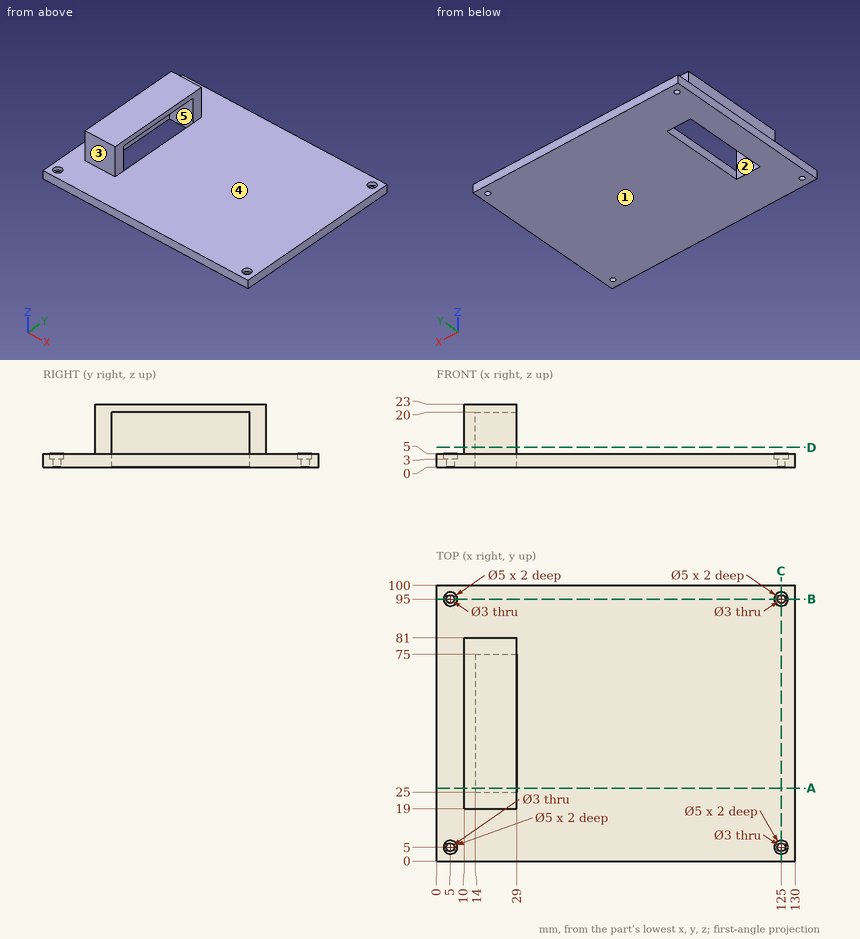
The drawing under review shows one solid part. Ordinate dimensions are in mm from its lowest x, y, z. A direction names the side the tool comes from. Give positions to 0.01 mm unless a question says otherwise; leave off trailing zeros. Order: outer loops, then holes, each group sorted by start corner. A loop starts at its lowest first (then second) coordinate and runs counter-clockwise, first axis right, second up. Notation, with made-up numbers: (52, -24) - (109, -24) arc R21 ccw to (109, 0) - close; hole circle Ø2 at (-36, -6.75). An arc over 180 degrees is marked (long way). Answer as a JSON object with one key per item and string values. Group by question number.
Item 1: Draft analysis for pull direction X (two halves, no side actions). For the marked faces 4 and 5, state which applies: pulls with the +X half, pulls with the -X half, needs draft (parallel to the pull), parting line crosses it, or undercut.
Item 2: Wall thickness on line 1 along Y through (x, z) = (5, 4.1); line 2 along Y through (x, z) = (125, 0.9); line 3 along X through (y, z) = (43, 3.25): over which ranges is each line inside the solid? List them lowest first.
Item 3: Take a section at A-A on y = 26.5. Give the boundary of the cut face in (x, z), and give its area (3 significant figures).
Item 4: Machinability: for the marked faces 1, 2 and 3, which of the approach directions +Z, -Z, +X, -X, +Y, -Y give a long, thin tool a straight path to every point of the face, cutting with its end or side? Answer none if there is none.
Item 5: Take a section at D-D on z = 7.25. Give the boundary of the cut face in (x, y), and give its area (3 significant figures).
Item 6: Take a section at C-C on x = 125. Give the boundary of the cut face in (y, z).
Item 7: Take a section at B-B on y = 95. Give the boundary of the cut face in (x, z), and give its area (3 significant figures).
Item 8: Clearance check with flat-ended pins moving along their axes: pin 1 Ø2.5 at (x, y) = (5, 5.5) entering from +Z; pin 2 Ø6 at (y, z) = (58, 8.5) entering from +X; pin 3 Ø1.5 at (y, z) = (47, 17) entering from -X. State where each tip first meets the part, or that it passes through.
Reported:
{
 "1": {"face 4": "needs draft", "face 5": "undercut"},
 "2": {"line 1": "0 to 2.5, 7.5 to 92.5, 97.5 to 100", "line 2": "0 to 3.5, 6.5 to 93.5, 96.5 to 100", "line 3": "0 to 14, 29 to 130"},
 "3": {"outline": "(0, 0) - (14, 0) - (14, 20) - (29, 20) - (29, 23) - (10, 23) - (10, 5) - (0, 5) - close; (29, 0) - (130, 0) - (130, 5) - (29, 5) - close", "area": "692 mm^2"},
 "4": {"face 1": "-Z, +X, -X, +Y, -Y", "face 2": "-Z", "face 3": "+Z, +X, -X, -Y"},
 "5": {"outline": "(10, 19) - (29, 19) - (29, 25) - (14, 25) - (14, 75) - (29, 75) - (29, 81) - (10, 81) - close", "area": "428 mm^2"},
 "6": {"outline": "(0, 0) - (3.5, 0) - (3.5, 3) - (2.5, 3) - (2.5, 5) - (0, 5) - close; (6.5, 0) - (93.5, 0) - (93.5, 3) - (92.5, 3) - (92.5, 5) - (7.5, 5) - (7.5, 3) - (6.5, 3) - close; (96.5, 0) - (100, 0) - (100, 5) - (97.5, 5) - (97.5, 3) - (96.5, 3) - close"},
 "7": {"outline": "(0, 0) - (3.5, 0) - (3.5, 3) - (2.5, 3) - (2.5, 5) - (0, 5) - close; (6.5, 0) - (123.5, 0) - (123.5, 3) - (122.5, 3) - (122.5, 5) - (7.5, 5) - (7.5, 3) - (6.5, 3) - close; (126.5, 0) - (130, 0) - (130, 5) - (127.5, 5) - (127.5, 3) - (126.5, 3) - close", "area": "612 mm^2"},
 "8": {"pin 1": "z = 3", "pin 2": "x = 14", "pin 3": "x = 10"}
}
